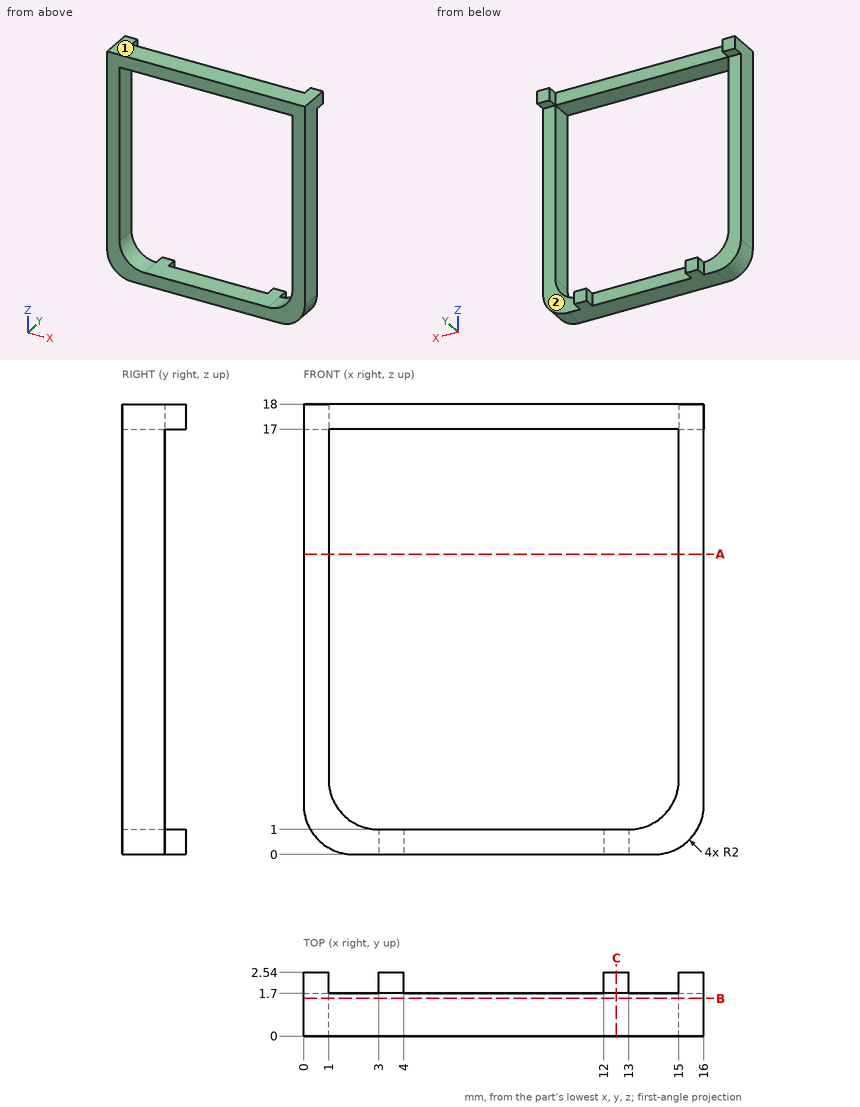
For this review, use the dimensioned drawing (mm, ordinates from the lowest corner) and the shaded views. A direction names the side the tool comes from. Round coordinates to 2 decimals unless told otherwise and drop trailing zeros. Write each loop counter-clockwise with the first axis right and the second up, starting at its lowest first coordinate (ties: lowest second). Pieces come first, ordered by that corner, then holes. Notation, with made-up numbers: M -39.5,19 L 17.5,19 A16 cw 17.5,26 Z; hole C -18,27.5 d9. An arc over 180 degrees is marked long. Write item = value, one per line. Start each with the question number.
(1) We need section B-B (y = 1.5). Give the boundary of the cut face in (x, z).
(2) We need section C-C (x = 12.5). Give the boundary of the cut face in (y, z).
(3) We need section A-A (z = 12). Give the boundary of the cut face in (x, y), then the cut area to 3 significant figures.
(4) Clearance check with flat-ended pins moving along their axes: pin 1 Ø0.9 at (x, z) = (1.5, 10.5) entering from +Y; pin 2 Ø0.8 at (x, z) = (6.5, 0.5) entering from +Y; pin 3 Ø0.9 at (y, z) = (2, 0.5) entering from -X; pin 4 Ø0.9 at (y, z) = (2, 0.5) entering from +X. State where each tip first meets the part, or that it passes through.
(5) For the marked faces 1 and 2, list the 3-axis set-ups (+Z, -Z, +X, -X, +Y, -Y) from which the entire face can be reached by the end or side of a thin tool; tool diameter is ignored.
(6) For line 1 along X through (y, z) = (0.35, 3); line 2 along Z through (x, y) = (10.75, 0.5); line 3 along Y through (x, z) = (15.25, 11.5), list the stretches that pass through material, from the lowest coordinate up.
Results found:
q1.outline = M 0,2 A2 ccw 2,0 L 14,0 A2 ccw 16,2 L 16,18 L 0,18 Z; hole M 1,3 A2 ccw 3,1 L 13,1 A2 ccw 15,3 L 15,17 L 1,17 Z
q2.outline = M 0,0 L 2.54,0 L 2.54,1 L 0,1 Z; M 0,17 L 1.7,17 L 1.7,18 L 0,18 Z
q3.outline = M 0,0 L 1,0 L 1,1.7 L 0,1.7 Z; M 15,0 L 16,0 L 16,1.7 L 15,1.7 Z
q3.area = 3.40 mm²
q4.pin_1 = through
q4.pin_2 = 1.7
q4.pin_3 = 0.37
q4.pin_4 = 15.63
q5.face_1 = +Z, +X, -X, +Y, -Y
q5.face_2 = -Z, +X, +Y
q6.line_1 = 0 to 1, 15 to 16
q6.line_2 = 0 to 1, 17 to 18
q6.line_3 = 0 to 1.7
